The figure shows three views and two pictorial views of one solid part (mm, origin at its lowest corner). Answer the questions. A direction names the side the tool comes from. Give positions to 0.01 mm unless a question says otherwise; leave off trailing zeros. Loops run counter-clockwise (first coordinate to the right, second up) from the corner with the lowest first, then second, coordinate; pieces in that order, holes last.
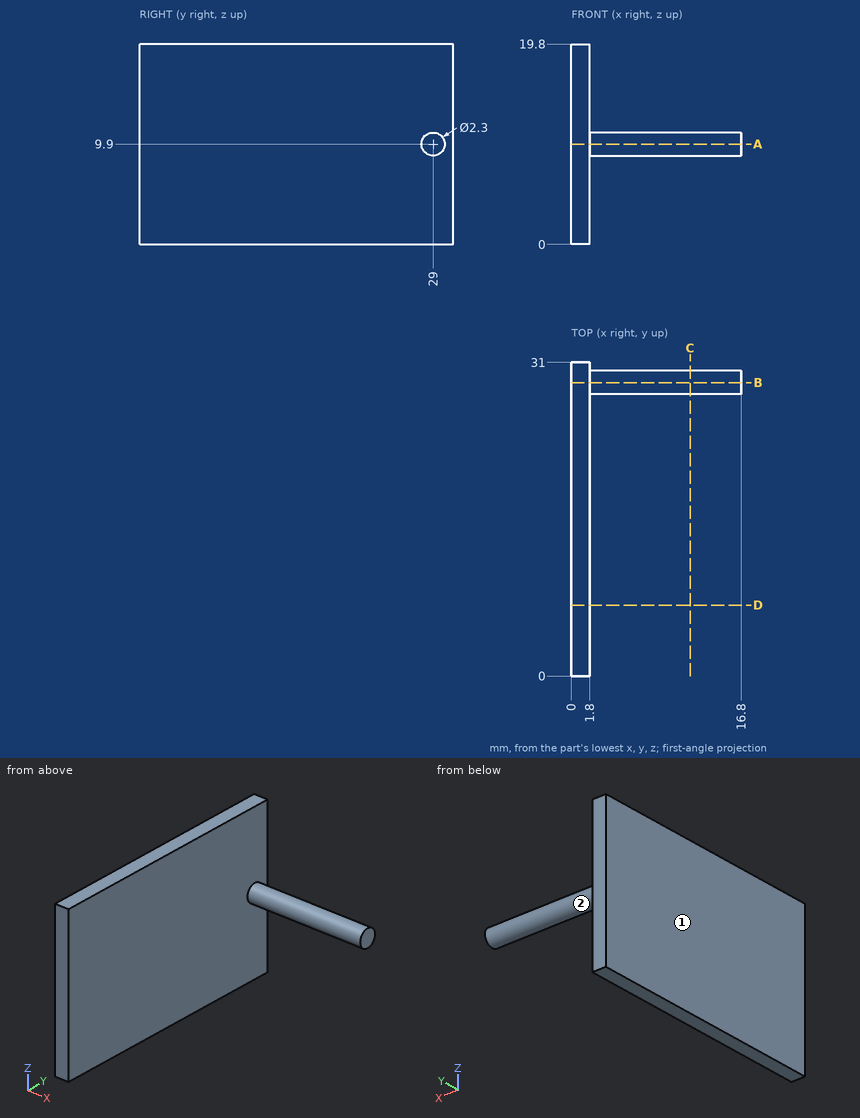
Q1. Given pin 1 (1 mm diameter, centred on y = 7, z = 6, fed in from +X); pin 2 (4 mm diameter, centred on x = 11, z = 6, fed in from +Y); pin 3 (8 mm diameter, centred on x = 7, z = 6.5, fed in from -Y), each flat-ended and moving along its own axis, determine where each tip first touches the part or whether it passes through.
Q2. Section A-A on z = 9.9 is taken. Give the vertices of the cut face in (x, y).
Q3. Section B-B on y = 29 is taken. Give the vertices of the cut face in (x, z).
Q4. Section D-D on y = 7 is taken. Give the vertices of the cut face in (x, z), plus the area to 3 significant figures.
Q5. Consider line 1 along X through (y, z) = (5, 15.25); line 2 along Y through (x, z) = (4.25, 10.75). Determine where each line is inside the solid, lowest interval first.
Q6. Which of the six approach directions +Z, -Z, +X, -X, +Y, -Y give full straight-line access (tool end or side, diameter ignored) to the marked faces 1 and 2?
Q7. Section C-C on x = 11.75 is taken. Give the vertices of the cut face in (y, z).
Check result:
1. pin 1: stops at x = 1.8
1. pin 2: passes through
1. pin 3: stops at y = 27.85
2. outline: (0, 0) - (1.8, 0) - (1.8, 27.85) - (16.8, 27.85) - (16.8, 30.15) - (1.8, 30.15) - (1.8, 31) - (0, 31) - close
3. outline: (0, 0) - (1.8, 0) - (1.8, 8.75) - (16.8, 8.75) - (16.8, 11.05) - (1.8, 11.05) - (1.8, 19.8) - (0, 19.8) - close
4. outline: (0, 0) - (1.8, 0) - (1.8, 19.8) - (0, 19.8) - close
4. area: 35.6 mm2
5. line 1: x = 0 to 1.8
5. line 2: y = 28.23 to 29.77
6. face 1: +Z, -Z, -X, +Y, -Y
6. face 2: +X
7. outline: circle Ø2.3 at (29, 9.9)
